Check sheet for the modelled part. Datum: model origin and axes. Units: mm. A direction names the side the tool comes from. Give positions to 0.01 mm unless a question says otherwise; leave off trailing zeros. Loops run counter-clockwise (first coordinate to the right, second up) from the corner with the lowest first, then second, coordinate; pieces in that order, holes last. Notation, with made-up numbers: (43.25, -31) -> (49.25, -31) arc R15 ccw to (49.25, -25) -> close; hole circle Ø9 at (49, 67). An arc over 180 degrees is marked (long way). Write each question's results on one line, items separated by ' | '. Start each with the question number.
Item 1: Cross-section at C-C on y = 9.5. Enter the section's corners in (x, z).
Item 2: Cross-section at B-B on z = -15.25. Enter the section's corners in (x, y) (1 decimal), then the cut area to 3 significant figures.
Item 3: Cross-section at A-A on x = 13.25. Enter the section's corners in (y, z) (3 decimals), then the cut area to 3 significant figures.
Item 4: Scan lines: line 1 along Y through (x, z) = (6.75, -25); line 2 along Z through (x, y) = (12, 13.25) (3 decimals); line 3 along X through (y, z) = (13.25, -17.5) (3 decimals). Record each from-to range of solid material in increasing order.
Item 5: Access from +Z, -Z, +X, -X, +Y, -Y to the whole of each face (thin tool, end or side, straight path). Record for faces 1 (the face through (10.125, 13, -15)), 2 (the face through (16.375, 13, -15)), 3 (the face through (0, 2, -15)), 4 (the face through (13, 13, -11.875)), 5 (the face through (13, 13, -18.125)).
Item 6: Gauge pin test, flat ends, axial feed: pin 1 Ø1.6 at (y, z) = (12.5, -16) entering from +X; pin 2 Ø6 at (y, z) = (5.5, -15) entering from +X; pin 3 Ø1.6 at (x, y) = (13.5, 12.5) entering from -Z; pin 4 Ø0.8 at (y, z) = (12.5, -14.5) entering from -X (3 decimals). Record the tip position at first contact, or that the pin passes through.
Item 7: Cross-section at D-D on x = 20.75. Enter the section's corners in (y, z).
from build123d import *

# Parameters (mm, degrees)
SKETCH1_W                = 240
SKETCH1_H                = 30
SKETCH1_W_2              = 6.25
SKETCH1_H_2              = 6.25
BOSS_EXTRUDE1_DEPTH      = 4
SKETCH2_W                = 6.25
SKETCH2_H                = 6.25
BOSS_EXTRUDE2_DEPTH      = 10.5
BOSS_EXTRUDE2_DEPTH_BACK = 4
SKETCH3_W                = 222.243091979
SKETCH3_H                = 95.437848018
CUT_EXTRUDE1_DEPTH       = 11.5
CUT_EXTRUDE1_DEPTH_BACK  = 5
FILLET1_R                = 1
CHAMFER1_SIZE            = 0.4
CHAMFER1_SIZE2           = 8


with BuildPart() as part:
    # Sketch1 → Boss-Extrude1 (new body)
    with BuildSketch(Plane(origin=(0, 0, 0), x_dir=(1, 0, 0), z_dir=(0, 1, 0))):
        with Locations((120, 15)):
            Rectangle(SKETCH1_W, SKETCH1_H)
        with Locations((13.25, 15)):
            Rectangle(SKETCH1_W_2, SKETCH1_H_2, mode=Mode.SUBTRACT)
        with Locations((43.75, 15)):
            Rectangle(SKETCH1_W_2, SKETCH1_H_2, mode=Mode.SUBTRACT)
        with Locations((74.25, 15)):
            Rectangle(SKETCH1_W_2, SKETCH1_H_2, mode=Mode.SUBTRACT)
        with Locations((104.75, 15)):
            Rectangle(SKETCH1_W_2, SKETCH1_H_2, mode=Mode.SUBTRACT)
        with Locations((135.25, 15)):
            Rectangle(SKETCH1_W_2, SKETCH1_H_2, mode=Mode.SUBTRACT)
        with Locations((165.75, 15)):
            Rectangle(SKETCH1_W_2, SKETCH1_H_2, mode=Mode.SUBTRACT)
        with Locations((196.25, 15)):
            Rectangle(SKETCH1_W_2, SKETCH1_H_2, mode=Mode.SUBTRACT)
        with Locations((226.75, 15)):
            Rectangle(SKETCH1_W_2, SKETCH1_H_2, mode=Mode.SUBTRACT)
    extrude(amount=BOSS_EXTRUDE1_DEPTH)

    # Sketch2 → Boss-Extrude2 (add, two sides)
    with BuildSketch(Plane(origin=(0, 4, 0), x_dir=(1, 0, 0), z_dir=(0, 1, 0))) as boss_extrude2_sk:
        with Locations((13.25, 15)):
            Rectangle(SKETCH2_W, SKETCH2_H)
        with Locations((43.75, 15)):
            Rectangle(SKETCH2_W, SKETCH2_H)
        with Locations((74.25, 15)):
            Rectangle(SKETCH2_W, SKETCH2_H)
        with Locations((104.75, 15)):
            Rectangle(SKETCH2_W, SKETCH2_H)
        with Locations((135.25, 15)):
            Rectangle(SKETCH2_W, SKETCH2_H)
        with Locations((165.75, 15)):
            Rectangle(SKETCH2_W, SKETCH2_H)
        with Locations((196.25, 15)):
            Rectangle(SKETCH2_W, SKETCH2_H)
        with Locations((226.75, 15)):
            Rectangle(SKETCH2_W, SKETCH2_H)
    extrude(amount=BOSS_EXTRUDE2_DEPTH)
    extrude(boss_extrude2_sk.sketch, amount=-BOSS_EXTRUDE2_DEPTH_BACK)

    # Sketch3 → Cut-Extrude1 (cut, two sides)
    with BuildSketch(Plane(origin=(0, 4, 0), x_dir=(1, 0, 0), z_dir=(0, 1, 0))) as cut_extrude1_sk:
        with Locations((133.951037232, 10.683129124)):
            Rectangle(SKETCH3_W, SKETCH3_H)
    extrude(amount=CUT_EXTRUDE1_DEPTH, mode=Mode.SUBTRACT)
    extrude(cut_extrude1_sk.sketch, amount=-CUT_EXTRUDE1_DEPTH_BACK, mode=Mode.SUBTRACT)

    # Fillet1
    fillet1_edges = [part.edges().sort_by_distance(p)[0] for p in [
        (10.125, 14.5, -15),
        (13.25, 14.5, -11.875),
        (16.375, 14.5, -15),
        (13.25, 14.5, -18.125),
    ]]
    fillet(fillet1_edges, radius=FILLET1_R)

    # Chamfer1
    chamfer1_edges = [part.edges().sort_by_distance(p)[0] for p in [
        (10.125, 4, -15),
        (13.25, 4, -11.875),
        (16.375, 4, -15),
        (13.25, 4, -18.125),
    ]]
    chamfer1_side = [part.faces().sort_by_distance(p)[0] for p in [
        (0.376986163, 4, -15),
    ]]
    chamfer(chamfer1_edges, length=CHAMFER1_SIZE, length2=CHAMFER1_SIZE2, reference=chamfer1_side[0])


solid = part.part
Answer sheet:
1) outline: (10, -18.25) -> (16.5, -18.25) -> (16.5, -11.75) -> (10, -11.75) -> close
2) outline: (0, 0) -> (22.8, 0) -> (22.8, 4) -> (16.8, 4) -> (16.4, 12) -> (16.4, 13.5) arc R1 ccw to (15.4, 14.5) -> (11.1, 14.5) arc R1 ccw to (10.1, 13.5) -> (10.1, 12) -> (9.7, 4) -> (0, 4) -> close | area: 160 mm²
3) outline: (0, -30) -> (4, -30) -> (4, -18.525) -> (12, -18.125) -> (13.5, -18.125) arc R1 ccw to (14.5, -17.125) -> (14.5, -12.875) arc R1 ccw to (13.5, -11.875) -> (12, -11.875) -> (4, -11.475) -> (4, 0) -> (0, 0) -> close | area: 188 mm²
4) line 1: y = 0 to 4 | line 2: z = -18.125 to -11.875 | line 3: x = 10.125 to 16.375
5) face 1: +Z, -Z, -X, +Y | face 2: +Z, -Z, +X, +Y | face 3: +Z, -Z, -X, +Y, -Y | face 4: +Z, +X, -X, +Y | face 5: -Z, +X, -X, +Y
6) pin 1: stops at x = 16.39 | pin 2: stops at x = 22.83 | pin 3: stops at z = -18.14 | pin 4: stops at x = 10.125
7) outline: (0, -30) -> (4, -30) -> (4, 0) -> (0, 0) -> close
